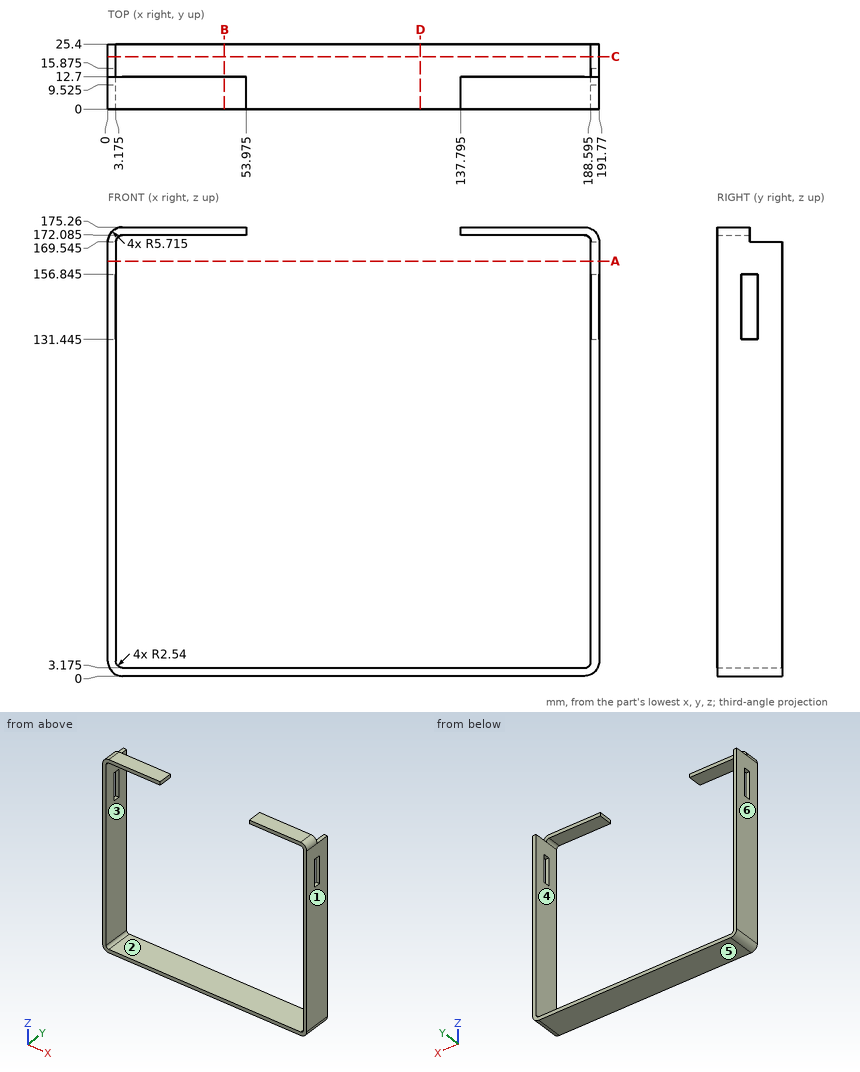
Drawing for the job (mm, zero at the part's lowest x, y, z). A direction names the side the tool comes from. Give positions to 0.01 mm unless a question says otherwise; leave off trailing zeros. Order: outer loops, then holes, each group sorted by start corner. A loop starts at its lowest first (then second) coordinate and runs counter-clockwise, first axis right, second up. Notation, with made-up numbers: M -32,66 L -28,66 A18 cw -28,94 Z; hole C -13,23.25 d9. An arc over 180 degrees is marked long. Write item = value, one per line. Start each with the question number.
(1) Slice it at A-A on z = 162. Write the cut outline in (x, y) (3 decimals), plus the area to 3 significant figures.
(2) Two-plate mould, pull along Z, no slides. Class the marked faces 3, 4, 5 and 6: released by +Z, released by -Z, zero draft, split by the parting line, or undercut.
(3) Slice it at D-D on x = 122. Write the cut outline in (y, z) (3 decimals), plus the area to 3 significant figures.
(4) Slice it at B-B on x = 45.5. Write the cut outline in (y, z) (3 decimals).
(5) Which spindle directions (+Z, -Z, +X, -X, +Y, -Y) get a long thin tool onto all of the face, cutting with end or side? Do the marked faces 1 and 2. Say none if no direction does.
(6) Slice it at C-C on y = 20.5. Write the cut outline in (x, z) (3 decimals).
(7) Probe L1, parallel to X at y = 10.5, z = 70 (3 decimals); L2, parallel to Z at x = 158.5, y = 10.25 (3 decimals); L3, parallel to Z at x = 76.5, y = 1.75 (3 decimals). List the from-to ranges inside material, lowest first. Write a range as [from, to].
(8) Pin check, flat tips, straight feed: pin 1 Ø2.5 at (y, z) = (4.5, 174) entering from -X; pin 2 Ø6.5 at (x, z) = (29, 171) entering from +Y; pin 3 Ø3.5 at (x, y) = (190.5, 11.5) entering from -Z. Stop position of each tip, or through.
Responses:
q1.outline = M 0,0 L 3.175,0 L 3.175,25.4 L 0,25.4 Z; M 188.595,0 L 191.77,0 L 191.77,25.4 L 188.595,25.4 Z
q1.area = 161 mm2
q2.face_3 = undercut
q2.face_4 = undercut
q2.face_5 = released by -Z
q2.face_6 = zero draft
q3.outline = M 0,0 L 25.4,0 L 25.4,3.175 L 0,3.175 Z
q3.area = 80.6 mm2
q4.outline = M 0,0 L 25.4,0 L 25.4,3.175 L 0,3.175 Z; M 0,172.085 L 12.7,172.085 L 12.7,175.26 L 0,175.26 Z
q5.face_1 = +Z, -Z, +X, +Y, -Y
q5.face_2 = +Y, -Y
q6.outline = M 0,5.715 A5.715 ccw 5.715,0 L 186.055,0 A5.715 ccw 191.77,5.715 L 191.77,169.545 L 188.595,169.545 L 188.595,5.715 A2.54 cw 186.055,3.175 L 5.715,3.175 A2.54 cw 3.175,5.715 L 3.175,169.545 L 0,169.545 Z
q7.L1 = [0, 3.175], [188.595, 191.77]
q7.L2 = [0, 3.175], [172.085, 175.26]
q7.L3 = [0, 3.175]
q8.pin_1 = 0.98
q8.pin_2 = 12.7
q8.pin_3 = 0.68
